from build123d import *

# Parameters (mm, degrees)
F3_DEPTH = 5
F4_DEPTH = 5
F5_COUNT = 14
F6_R     = 0.925
F7_DEPTH = 5.001


with BuildPart() as f3:
    # F1 (on Top) → F3 (new body)
    with BuildSketch(Plane.XY):
        with BuildLine():
            ThreePointArc((-0.4153368417, 2.9807568553), (-1.9757830613, -2.2701756357), (3.0095541401, 0))
            ThreePointArc((3.0095541401, 0), (2.2701756357, 1.9757830613), (0.4153368417, 2.9807568553))
            ThreePointArc((0.4153368417, 2.9807568553), (0.2081669857, 3.0023461873), (0, 3.0095541401))
            ThreePointArc((0, 3.0095541401), (-0.2081669857, 3.0023461873), (-0.4153368417, 2.9807568553))
        make_face()
    extrude(amount=F3_DEPTH)

    # F1 (on Top) → F4 (join)
    with BuildSketch(Plane.XY):
        with BuildLine():
            ThreePointArc((0, 3.0095541401), (0.2081669857, 3.0023461873), (0.4153368417, 2.9807568553))
            Line((0.4153368417, 2.9807568553), (0.208250893, 4.2702265482))
            ThreePointArc((0.208250893, 4.2702265482), (0.1041563607, 4.2740325993), (0, 4.2753015341))
            ThreePointArc((0, 4.2753015341), (-0.1041563607, 4.2740325993), (-0.208250893, 4.2702265482))
            Line((-0.208250893, 4.2702265482), (-0.4153368417, 2.9807568553))
            ThreePointArc((-0.4153368417, 2.9807568553), (-0.2081669857, 3.0023461873), (0, 3.0095541401))
        make_face()
    extrude(amount=F4_DEPTH)

    # F5: F3 ×14 about axis
    f5_axis = Axis((0, 0, 3.5011740401), (0, 0, -1))


with BuildPart() as f3_1:
    add(f3.part)
    for i in range(1, F5_COUNT):
        add(f3.part.rotate(f5_axis, i * 360 / F5_COUNT))

    # F6 (on face) → F7 (cut, through all)
    with BuildSketch(Plane.XY.offset(5)):
        Circle(F6_R)
    extrude(amount=-F7_DEPTH, mode=Mode.SUBTRACT)


solid = f3_1.part
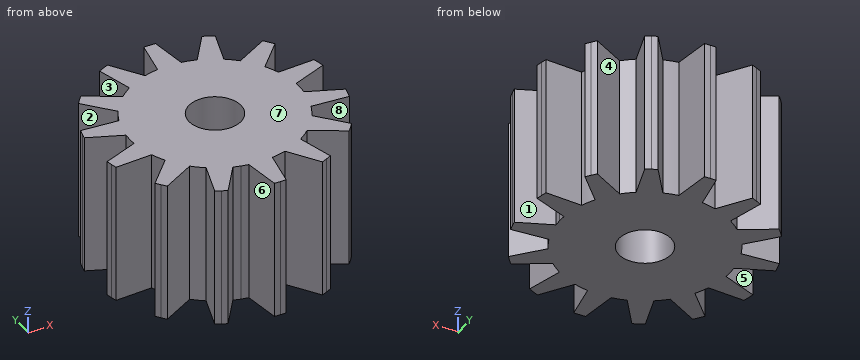
Work out the finished part from the listing and answer in its coordinate system (mm). Face numbers are marked on the shaded views. A direction names the side the tool comes from. Coordinates: 2 decimals unless noted, no trailing zeros. Loops run counter-clockwise (first coordinate to the right, second up) from the corner with the lowest first, then second, coordinate; pieces in that order, holes last. Notation, with made-up numbers: (21.5, -7.75) -> (35.5, -7.75) arc R27 cw to (35.5, 28.25) -> close; hole circle Ø5 at (58, 48). An arc over 180 degrees is marked (long way). Answer as CSV lines item,"result".
1) For the marked faces 4, 5, 6, 7 and 8, determine the directions among +Z, -Z, +X, -X, +Y, -Y from which every point of the face is accessible in a straight line to the end or side of a thin tool.
A:
face 4,"+Z, -Z, +Y"
face 5,"+Z, -Z, -X"
face 6,"+Z, -Z, -Y"
face 7,"+Z, +X, -X, +Y, -Y"
face 8,"+Z, -Z"
2) For a pull along X with two mould halves and no side action, classify the marked faces 1, 2 and 3 as released by +X, released by -X, zero draft, split by the parting line, or undercut.
A:
face 1,"released by +X"
face 2,"released by -X"
face 3,"undercut"
3) Flat-ended cylindrical pins translate along their axes: pin 1 (1 mm diameter, centred on x = -1.5, z = 4, fed in from -Y); pin 2 (1.5 mm diameter, centred on y = -2.5, z = 2.5, fed in from -X). Find the tip coordinate at first contact, or state that the pin passes through.
A:
pin 1,"stops at y = -3.94"
pin 2,"stops at x = -3.47"
4) The part is cut by section B-B (x = 2.25). Give the vertices of the cut face in (y, z).
A:
outline,"(-2.28, 0) -> (2.28, 0) -> (2.28, 5) -> (-2.28, 5) -> close"
5) The part is cut by section A-A (y = -3.5). Give the vertices of the cut face in (x, z).
A:
outline,"(-1.96, 0) -> (-1.36, 0) -> (-1.36, 5) -> (-1.96, 5) -> close; (-0.33, 0) -> (0.33, 0) -> (0.33, 5) -> (-0.33, 5) -> close; (1.36, 0) -> (1.96, 0) -> (1.96, 5) -> (1.36, 5) -> close"
6) The part is cut by section C-C (y = 2). Give the vertices of the cut face in (x, z).
A:
outline,"(-3.01, 0) -> (3.01, 0) -> (3.01, 5) -> (-3.01, 5) -> close"
7) Straight lines are drawn through the part: probe 1 along X at (y, z) = (-2.25, 1.55); probe 2 along Y at (x, z) = (3.25, 1.7); probe 3 along X at (y, z) = (2.75, 1.7). For each, find the intervals that lie inside material, in ascending order.
A:
probe 1,"x = -3.24 to -2.19, -2 to 2, 2.19 to 3.24"
probe 2,"y = -2.78 to -2.26, -1.1 to -0.36, 0.36 to 1.1, 2.26 to 2.78"
probe 3,"x = -3.27 to -3.08, -1.74 to 1.74, 3.08 to 3.27"
